Autodesk Inventor part; units mm, degrees
ref_plane "YZ Plane" through (0, 0, 0) normal (1, 0, 0) x (0, 1, 0)
ref_plane "XZ Plane" through (0, 0, 0) normal (0, 1, 0) x (-1, 0, 0)
ref_plane "XY Plane" through (0, 0, 0) normal (0, 0, 1) x (1, 0, 0)
sketch "Эскиз1" plane through (0, 0, 0) normal (0, 0, 1) x (1, 0, 0)
  line L0 (-14.25, 29.75) -> (14.25, 29.75)
  line L1 (14.25, 29.75) -> (14.25, -29.75)
  line L2 (14.25, -29.75) -> (-14.25, -29.75)
  line L3 (-14.25, -29.75) -> (-14.25, 29.75)
  line L4 (0, -41.65) -> (0, 41.65)
  line L5 (-19.95, 0) -> (19.95, 0)
  line L6 (-12.25, 27.75) -> (12.25, 27.75)
  line L7 (12.25, 27.75) -> (12.25, -27.75)
  line L8 (12.25, -27.75) -> (-12.25, -27.75)
  line L9 (-12.25, -27.75) -> (-12.25, 27.75)
  point P0 (0, 0)
  dimension "d0" = 28.5
  dimension "d1" = 59.5
  dimension "d2" = 2
extrude "Выдавливание1" add sketch "Эскиз1" along normal blind 2 contours L0 L4 L6 L9 L5 L3 | L0 L1 L5 L7 L6 L4 | L5 L9 L8 L4 L2 L3 | L1 L2 L4 L8 L7 L5
sketch "Эскиз2" plane through (0, 0, 2) normal (0, 0, 1) x (1, 0, 0)
  line L0 (-16.25, 31.5) -> (16.25, 31.5)
  line L1 (16.25, 31.5) -> (16.25, -31.5)
  line L2 (16.25, -31.5) -> (-16.25, -31.5)
  line L3 (-16.25, -31.5) -> (-16.25, 31.5)
  line L4 (0, -44.1) -> (0, 44.1)
  line L5 (-22.75, 0) -> (22.75, 0)
  point P0 (0, 0)
  dimension "d5" = 63
  dimension "d6" = 32.5
extrude "Выдавливание2" add sketch "Эскиз2" along normal blind 1.5
sketch "Эскиз3" plane through (0, 0, 2) normal (0, 0, -1) x (-1, 0, 0)
  line L0 (15, -30.5) -> (-15, -30.5)
  line L1 (-15, -30.5) -> (-15, 30.5)
  line L2 (-15, 30.5) -> (15, 30.5)
  line L3 (15, 30.5) -> (15, -30.5)
  line L4 (0, -44.1) -> (0, 44.1)
  line L5 (22.75, 0) -> (-22.75, 0)
  line L6 (14.25, -29.75) -> (-14.25, -29.75)
  line L7 (1.6881, -30.5) -> (-1.7436, -30.5)
  line L8 (-1.7436, -30.5) -> (-1.7436, -29.75)
  line L9 (-1.7436, -29.75) -> (1.6881, -29.75)
  line L10 (1.6881, -29.75) -> (1.6881, -30.5)
  line L11 (1.6881, 29.75) -> (-1.8544, 29.75)
  line L12 (-1.8544, 29.75) -> (-1.8544, 30.5)
  line L13 (-1.8544, 30.5) -> (1.6881, 30.5)
  line L14 (1.6881, 30.5) -> (1.6881, 29.75)
  line L15 (14.25, 29.75) -> (14.25, -29.75)
  line L16 (15, 22.8864) -> (14.25, 22.8864)
  line L17 (14.25, 22.8864) -> (14.25, 25.9613)
  line L18 (14.25, 25.9613) -> (15, 25.9613)
  line L19 (15, 25.9613) -> (15, 22.8864)
  line L20 (15, -24.3425) -> (14.25, -24.3425)
  line L21 (14.25, -24.3425) -> (14.25, -20.2031)
  line L22 (14.25, -20.2031) -> (15, -20.2031)
  line L23 (15, -20.2031) -> (15, -24.3425)
  line L24 (-14.2166, -25.1255) -> (-15, -25.1255)
  line L25 (-15, -25.1255) -> (-15, -18.943)
  line L26 (-15, -18.943) -> (-14.2166, -18.943)
  line L27 (-14.2166, -18.943) -> (-14.2166, -25.1255)
  line L28 (-14.2166, 21.6162) -> (-15, 21.6162)
  line L29 (-15, 21.6162) -> (-15, 25.9613)
  line L30 (-15, 25.9613) -> (-14.2166, 25.9613)
  line L31 (-14.2166, 25.9613) -> (-14.2166, 21.6162)
  point P0 (0, 0)
  point P1 (0, 29.75)
  point P2 (0, 30.5)
  point P3 (1.6881, -29.75)
  dimension "d9" = 61
  dimension "d10" = 30
extrude "Выдавливание3" add sketch "Эскиз3" along normal blind 2 contours L0 L4 L6 L10 | L20 L15 L22 L3 | L0 L8 L6 L4 | L16 L15 L18 L3 | L1 L26 L27 L24 | L11 L12 L2 L4 | L1 L30 L31 L28
sketch "Эскиз4" plane through (0, 0, 3.5) normal (0, 0, 1) x (1, 0, 0)
  circle A0 centre (0, -10) radius 3.25
  circle A1 centre (0, 10) radius 3.25
  line L0 (-22.75, 0) -> (22.75, 0)
  point P0 (0, 0)
  dimension "d13" = 6.5
  dimension "d14" = 6.5
  dimension "d15" = 20
extrude "Выдавливание4" cut sketch "Эскиз4" against normal blind 2
fillet "Сопряжение1" radius 2 4 edges at (-16.25, 31.5, 2.75) (16.25, 31.5, 2.75) (16.25, -31.5, 2.75) (-16.25, -31.5, 2.75)
sketch "Эскиз6" plane through (14.25, -18.943, 0) normal (1, 0, 0) x (0, 0, -1)
  line L0 (0, 40.5592) -> (-2, 40.5592)
  line L1 (-2, 0) -> (-2, 40.5592)
  line L2 (-2, 0) -> (0, 0)
  line L3 (0, 0) -> (0, 40.5592)
  point P0 (0, 18.943)
extrude "Выдавливание6" add sketch "Эскиз6" along normal up to surface (0.75 mm away)
sketch "Эскиз7" plane through (-14.25, -20.2031, 0) normal (-1, 0, 0) x (0, 0, 1)
  line L0 (0, 0) -> (2, 0)
  line L1 (2, 43.0894) -> (2, 0)
  line L2 (2, 43.0894) -> (0, 43.0894)
  line L3 (0, 43.0894) -> (0, 0)
  point P0 (0, 20.2031)
extrude "Выдавливание7" add sketch "Эскиз7" along normal up to surface (0.75 mm away)
properties part number "нижняя часть блока аккумов"
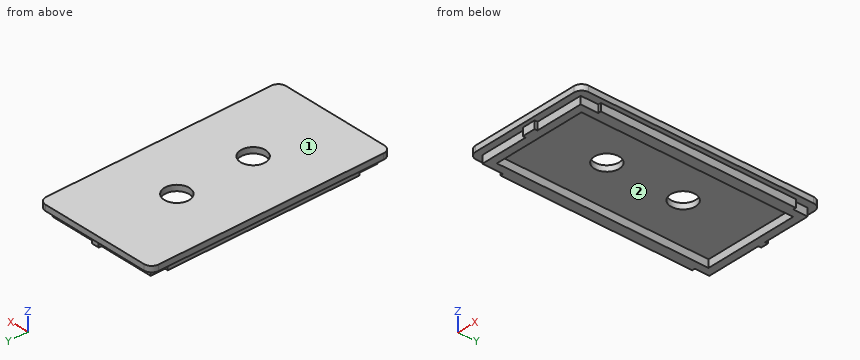
Design review of the part built by this model. Coordinates are the model's own, in mm. Face numbers are marked on the shaded views. Coordinates: 2 decimals unless noted, no trailing zeros. Order: outer loops, then holes, each group sorted by start corner. A loop starts at its lowest first (then second) coordinate and runs counter-clockwise, first axis right, second up.
1) Take a section at D-D, the plane x = -5. Give the boundary of the cut face in (y, z), and give its area (4 significant figures).
2) Take a section at B-B, the plane y = 10. Give the boundary of the cut face in (x, z), and give its area (3 significant figures).
3) Take a section at A-A, the plane z = 2.6. Give the boundary of the cut face in (x, y).
4) Take a section at C-C, the plane y = 21.5. Give the boundary of the cut face in (x, z).
5) Wall thickness on line 1 along Y through (x, z) = (0, 2.3); line 2 along Y through (x, z) = (1.5, 0.7); line 3 along X through (y, z) = (3.5, 1.35): over which ranges is each line inside the solid? List them lowest first.
6) Mouldability with a two-part tool opening along Y and no side actions: class the marked faces 1 and 2 as +Y half, -Y half, draft (parallel to the pull), parting line (faces both ways), or undercut.
7) Clearance check with flat-ended pins moving along their axes: pin 1 (0.8 mm diameter, centred on x = -15, z = 0.5, fed in from -Y); pin 2 (12 mm diameter, centred on x = -5.5, y = -13.5, fed in from -Z); pin 3 (5 mm diameter, centred on x = 0, y = -10, fed in from +Z); pin 4 (0.6 mm diameter, centred on y = 28, z = 1.5, fed in from +X). State where each tip first meets the part, or that it passes through.
Returned:
1. outline: (-31.5, 2) - (-29.75, 2) - (-29.75, 0) - (-27.75, 0) - (-27.75, 2) - (27.75, 2) - (27.75, 0) - (29.75, 0) - (29.75, 2) - (31.5, 2) - (31.5, 3.5) - (-31.5, 3.5) - close
1. area: 102.5 mm2
2. outline: (-16.25, 2) - (-15, 2) - (-15, 0) - (-12.25, 0) - (-12.25, 2) - (-3.25, 2) - (-3.25, 3.5) - (-16.25, 3.5) - close; (3.25, 2) - (12.25, 2) - (12.25, 0) - (15, 0) - (15, 2) - (16.25, 2) - (16.25, 3.5) - (3.25, 3.5) - close
2. area: 50.0 mm2
3. outline: (-16.25, -29.5) arc R2 ccw to (-14.25, -31.5) - (14.25, -31.5) arc R2 ccw to (16.25, -29.5) - (16.25, 29.5) arc R2 ccw to (14.25, 31.5) - (-14.25, 31.5) arc R2 ccw to (-16.25, 29.5) - close; hole circle Ø6.5 at (0, -10); hole circle Ø6.5 at (0, 10)
4. outline: (-16.25, 2) - (-15, 2) - (-15, 0) - (-12.25, 0) - (-12.25, 2) - (12.25, 2) - (12.25, 0) - (15, 0) - (15, 2) - (16.25, 2) - (16.25, 3.5) - (-16.25, 3.5) - close
5. line 1: y = -31.5 to -13.25, -6.75 to 6.75, 13.25 to 31.5
5. line 2: y = -30.5 to -27.75, 27.75 to 30.5
5. line 3: x = -15 to -12.25, 12.25 to 15
6. face 1: draft
6. face 2: undercut
7. pin 1: stops at y = -24.34
7. pin 2: stops at z = 2
7. pin 3: passes through
7. pin 4: stops at x = 14.25
